For this review, take the finished solid that the model builds, in its own axes (mm). A direction names the side the tool comes from. Coordinates: 2 decimals unless noted, no trailing zeros. Write each loop counter-clockwise with the first axis right and the second up, starting at its lowest first coordinate (ties: lowest second). Pieces come first, ordered by that corner, then holes. Notation, with made-up numbers: (-31, 37) -> (1, 37) arc R25 ccw to (1, 75) -> close; hole circle Ø5 at (31.5, -34.5). An arc over 180 degrees is marked (long way). One line per item, written item: value. Start each with the question number.
1) Add section A-A (x = 12.7). State the section outline as (y, z) points, and give its area (3 significant figures).
2) Mouldability with a two-part tool opening along X and no side actions: class faces 6 (the flat face through (33, -16, 22.112)), 7 (the flat face through (0, -9, 8)), 8 (the cylindrical face through (25.403, -15.735, 14.341)) as released by +X, released by -X, zero draft, split by the parting line, or undercut.
3) Add section C-C (z = 14.75). State the section outline as (x, y) points (3 decimals).
4) For probe 1 along Y at (x, z) = (12.7, 10.5); probe 2 along Z at (x, y) = (18.5, -1.75); probe 3 along Z at (x, y) = (22, -10.25), list the stretches that pass through material, from the lowest coordinate up. Write a range as from..to.
5) Add section D-D (x = 23.5). State the section outline as (y, z) points, and give its area (3 significant figures).
6) Machinability: for faces 1 (the flat face through (8, -9, 15.762)), 2 (the flat face through (7, -19.05, 10)), 3 (the flat face through (29, -6.35, 25)), 4 (the flat face through (3, -9, 0)), 5 (the flat face through (6.35, -9, 3)), which of the approach directions +Z, -Z, +X, -X, +Y, -Y give a long, thin tool a straight path to every point of the face, cutting with its end or side? Answer none if there is none.
7) For pin 1 Ø6 at (y, z) = (-5.5, 21.5) entering from -X; pin 2 Ø1 at (x, y) = (24.5, -22) entering from +Z; pin 3 Ø3 at (x, y) = (19.5, -22) entering from -Z, all flat-tipped, find the tip position at first contact; note any pin that passes through.
8) Add section B-B (y = -8). State the section outline as (x, z) points.
from build123d import *

# Parameters (mm, degrees)
F1_DEPTH = 19.05
F3_DEPTH = 6.35
F4_W     = 19.05
F4_H     = 6.35
F5_DEPTH = 38.101
F6_R     = 3.175
F7_DEPTH = 22.112613
F8_R     = 3.175
F9_DEPTH = 15.762613


with BuildPart() as f1:
    # F0 (on Front) → F1 (new body)
    with BuildSketch(Plane.XZ):
        Polygon((0, 15.761613), (0, 0), (6.35, 0), (6.35, 6.35), (38.1, 6.35), (38.1, 28.461613), (19.05, 28.461613), (19.05, 15.761613), align=None)
    extrude(amount=F1_DEPTH)

    # F2 (on face) → F3 (join)
    with BuildSketch(Plane.XZ.offset(19.05)):
        Polygon((38.1, 28.461613), (19.05, 28.461613), (19.05, 15.761613), (19.05, 6.35), (38.1, 6.35), align=None)
    extrude(amount=F3_DEPTH)

    # F4 (on face) → F5 (cut, through all)
    with BuildSketch(Plane.YZ.offset(38.1)):
        with Locations((-15.875, 25.286613)):
            Rectangle(F4_W, F4_H)
    extrude(amount=-F5_DEPTH, mode=Mode.SUBTRACT)

    # F6 (on face) → F7 (cut, through all)
    with BuildSketch(Plane.XY.offset(22.111613)):
        with Locations((28.575, -15.875)):
            Circle(F6_R)
    extrude(amount=-F7_DEPTH, mode=Mode.SUBTRACT)

    # F8 (on face) → F9 (cut, through all)
    with BuildSketch(Plane.XY.offset(15.761613)):
        with Locations((12.7, -9.398)):
            Circle(F8_R)
    extrude(amount=-F9_DEPTH, mode=Mode.SUBTRACT)


solid = f1.part
Numbers:
1. outline: (-19.05, 6.35) -> (-12.57, 6.35) -> (-12.57, 15.76) -> (-19.05, 15.76) -> close; (-6.22, 6.35) -> (0, 6.35) -> (0, 15.76) -> (-6.22, 15.76) -> close
1. area: 120 mm²
2. face 6: zero draft
2. face 7: released by -X
2. face 8: undercut
3. outline: (0, -19.05) -> (19.05, -19.05) -> (19.05, -25.4) -> (38.1, -25.4) -> (38.1, 0) -> (0, 0) -> close; hole circle Ø6.35 at (12.7, -9.398); hole circle Ø6.35 at (28.575, -15.875)
4. probe 1: -19.05..-12.57, -6.22..0
4. probe 2: 6.35..15.76
4. probe 3: 6.35..22.11
5. outline: (-25.4, 6.35) -> (0, 6.35) -> (0, 28.46) -> (-6.35, 28.46) -> (-6.35, 22.11) -> (-25.4, 22.11) -> close
5. area: 441 mm²
6. face 1: +Z, -X, +Y, -Y
6. face 2: +Z, -Z, -X, -Y
6. face 3: +Z, +X, -X, -Y
6. face 4: -Z, +X, -X, +Y, -Y
6. face 5: -Z, +X, +Y, -Y
7. pin 1: x = 19.05
7. pin 2: z = 22.11
7. pin 3: z = 6.35
8. outline: (0, 0) -> (6.35, 0) -> (6.35, 6.35) -> (9.85, 6.35) -> (9.85, 15.76) -> (0, 15.76) -> close; (15.55, 6.35) -> (38.1, 6.35) -> (38.1, 22.11) -> (19.05, 22.11) -> (19.05, 15.76) -> (15.55, 15.76) -> close
